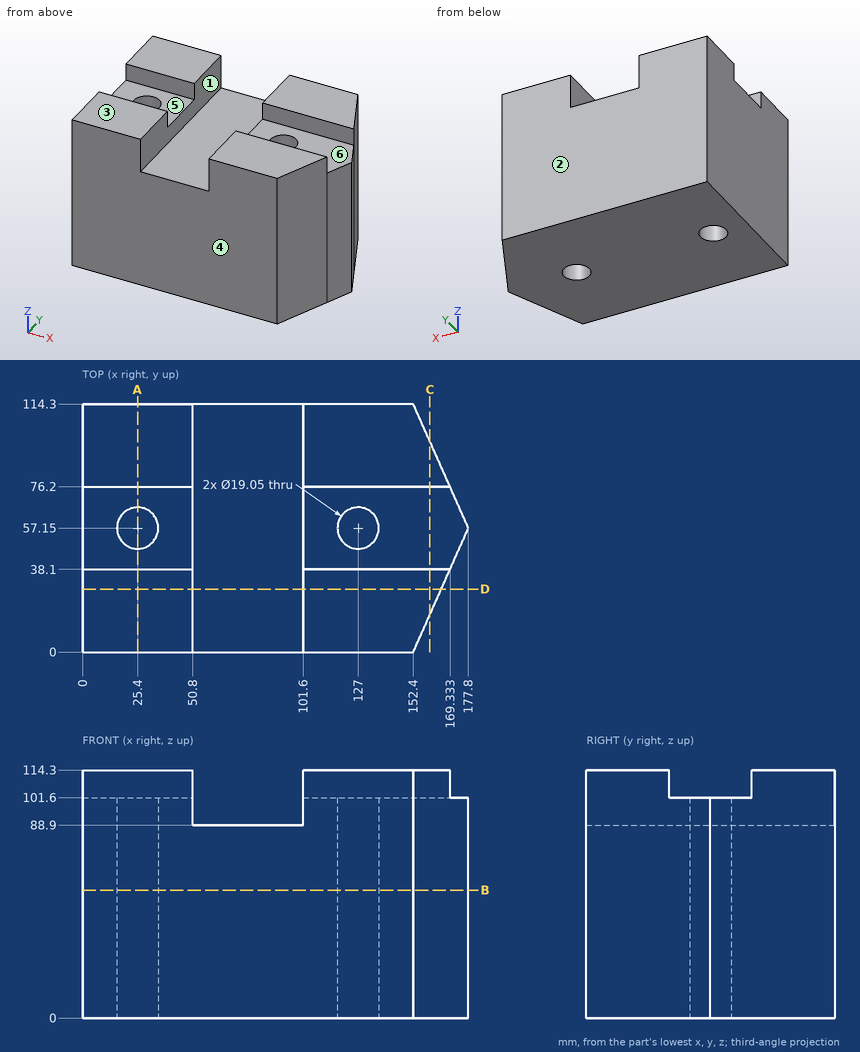
For this review, use the dimensioned drawing (mm, ordinates from the lowest corner) and the shaded views. A direction names the side the tool comes from. Coordinates: 2 decimals unless noted, no trailing zeros. Write each loop counter-clockwise with the first axis right and the second up, starting at its lowest first coordinate (ties: lowest second). Pieces come first, ordered by that corner, then holes. Notation, with made-up numbers: (-31.75, 13.5) - (-16.75, 13.5) arc R18 cw to (-16.75, 20.5) - close; hole circle Ø2 at (52.5, 59.25). An arc over 180 degrees is marked (long way). Answer as a JSON object with one key per item and string values. Group by question number.
1. Clearance check with flat-ended pins moving along their axes: pin 1 Ø1 at (y, z) = (103, 39.5) entering from +X (1 decimal); pin 2 Ø15 at (x, y) = (78, 74.5) entering from +Z; pin 3 Ø11.5 at (x, y) = (145.5, 53.5) entering from +Z; pin 4 Ø11.5 at (x, y) = (25.4, 57.15) entering from +Z. State where each tip first meets the part, or that it passes through.
2. Add section C-C (x = 160). Give the boundary of the cut face in (y, z), plus the area to 3 significant figures.
3. Mouldability with a two-part tool opening along Y and no side actions: class the marked faces 3, 4, 5 and 6 as pulls with the +Y half, pulls with the -Y half, needs draft (parallel to the pull), parting line crosses it, or undercut.
4. Add section D-D (y = 29). Give the boundary of the cut face in (x, z).
5. Machinability: for the marked faces 1 and 2, which of the approach directions +Z, -Z, +X, -X, +Y, -Y give a long, thin tool a straight path to every point of the face, cutting with its end or side? Answer none if there is none.
6. Add section A-A (x = 25.4). Give the boundary of the cut face in (y, z) (1 decimal), plus the area to 3 significant figures.
7. Add section B-B (z = 59). Give the number of separate pieces and of enclosed holes in the cut face, plus the area to 3 significant figures.
8. To check wall thickness, follow probe 1 along X at (y, z) = (57, 61) (1 decimal); probe 2 along Y at (x, z) = (144.5, 103); probe 3 along X at (y, z) = (65, 89) (1 decimal). State the ranges of each line that lie inside material, in increasing order.
Findings:
{
 "1": {"pin 1": "x = 157.6", "pin 2": "z = 88.9", "pin 3": "z = 101.6", "pin 4": "through"},
 "2": {"outline": "(17.1, 0) - (97.2, 0) - (97.2, 114.3) - (76.2, 114.3) - (76.2, 101.6) - (38.1, 101.6) - (38.1, 114.3) - (17.1, 114.3) - close", "area": "8,670 mm²"},
 "3": {"face 3": "needs draft", "face 4": "pulls with the -Y half", "face 5": "undercut", "face 6": "undercut"},
 "4": {"outline": "(0, 0) - (165.29, 0) - (165.29, 114.3) - (101.6, 114.3) - (101.6, 88.9) - (50.8, 88.9) - (50.8, 114.3) - (0, 114.3) - close"},
 "5": {"face 1": "+Z, +Y, -Y", "face 2": "+Z, -Z, +X, -X, +Y"},
 "6": {"outline": "(0, 0) - (47.6, 0) - (47.6, 101.6) - (38.1, 101.6) - (38.1, 114.3) - (0, 114.3) - close; (66.7, 0) - (114.3, 0) - (114.3, 114.3) - (76.2, 114.3) - (76.2, 101.6) - (66.7, 101.6) - close", "area": "10,600 mm²"},
 "7": {"separate pieces": "1", "enclosed holes": "2", "area": "18,300 mm²"},
 "8": {"probe 1": "0 to 15.9, 34.9 to 117.5, 136.5 to 177.7", "probe 2": "0 to 38.1, 76.2 to 114.3", "probe 3": "0 to 20, 30.8 to 50.8, 101.6 to 121.6, 132.4 to 174.3"}
}
